Model file for the job. Use its own axes, mm. A direction names the side the tool comes from. Round coordinates to 2 decimals unless told otherwise and drop trailing zeros. Loops run counter-clockwise (first coordinate to the right, second up) from the corner with the lowest first, then second, coordinate; pieces in that order, holes last. Notation, with made-up numbers: M 32,47.5 L 43,47.5 A13 cw 43,58.5 Z; hole C 59,-34 d8. An arc over 180 degrees is marked long. Answer in a Markdown table with one row per item.
from build123d import *

# Parameters (mm, degrees)
ESQUISSE1_R             = 8.5
BOSS_EXTRU_1_DEPTH      = 7
ESQUISSE2_W             = 6
ESQUISSE2_H             = 2.6
ENL_V_MAT_EXTRU_1_DEPTH = 14.910427743
ESQUISSE7_R             = 2.95
ENL_V_MAT_EXTRU_8_DEPTH = 21.087060672
ESQUISSE9_R             = 4
BOSS_EXTRU_2_DEPTH      = 7
ENL_V_MAT_EXTRU_9_DEPTH = 19.45264218


with BuildPart() as part:
    # Esquisse1 → Boss.-Extru.1 (new body)
    with BuildSketch(Plane.XY):
        Circle(ESQUISSE1_R)
    extrude(amount=BOSS_EXTRU_1_DEPTH)

    # Esquisse2 → Enlèv. mat.-Extru.1 (cut, through all)
    with BuildSketch(Plane(origin=(0, 0, 0), x_dir=(-1, 0, 0), z_dir=(0, 0, -1))):
        with Locations((0, 4)):
            Rectangle(ESQUISSE2_W, ESQUISSE2_H)
    extrude(amount=-ENL_V_MAT_EXTRU_1_DEPTH, mode=Mode.SUBTRACT)

    # Enlèv. mat.-Extru.2: read off the stored shape, not the designer's step
    # Enlèv. mat.-Extru.2 outline → Enlèv. mat.-Extru.2 (revolve, cut)
    with BuildSketch(Plane.XY.offset(3.5)):
        Polygon((0, 5.3), (1.554616831, 5.3), (1.498760014, 8.500034923), (0, 8.500034923), align=None)
        Polygon((1.6, 2.7), (0, 2.7), (0, 0.7), (1.56508987, 0.7), align=None)
    revolve(axis=Axis((0, 0, 3.5), (0, 1, 0)), mode=Mode.SUBTRACT)

    # Esquisse7 → Enlèv. mat.-Extru.8 (cut, through all)
    with BuildSketch(Plane(origin=(0, 8.3, 0), x_dir=(1, 0, 0), z_dir=(0, 1, 0))):
        with Locations((0, -3.5)):
            Circle(ESQUISSE7_R)
    extrude(amount=ENL_V_MAT_EXTRU_8_DEPTH, mode=Mode.SUBTRACT)

    # Chanfrein1: read off the stored shape, not the designer's step
    # Chanfrein1 outline → Chanfrein1 (revolve, cut)
    with BuildSketch(Plane.XY.offset(3.5)):
        Polygon((2.95, 6.747748364), (2.95, 8.3), (1.502251636, 8.3), (1.553718474, 5.351466838), align=None)
    revolve(axis=Axis((0, 0, 3.5), (0, 1, 0)), mode=Mode.SUBTRACT)

    # Esquisse9 → Boss.-Extru.2 (add)
    with BuildSketch(Plane.XY.offset(7)):
        with Locations(Location((0, -1, 0), (0, 0, 112.331645009))):
            Circle(ESQUISSE9_R)
    extrude(amount=BOSS_EXTRU_2_DEPTH)

    # Esquisse10 → Enlèv. mat.-Extru.9 (cut, through all)
    with BuildSketch(Plane(origin=(0, 0, 0), x_dir=(-1, 0, 0), z_dir=(0, 0, -1))):
        with BuildLine():
            Line((-1.549193338, 2.15), (1.549193338, 2.15))
            ThreePointArc((1.549193338, 2.15), (0, -2.65), (-1.549193338, 2.15))
        make_face()
    extrude(amount=-ENL_V_MAT_EXTRU_9_DEPTH, mode=Mode.SUBTRACT)


solid = part.part
1. Wall check: probe 1 along Z at (x, y) = (0, 7.6); probe 2 along Y at (x, z) = (0, 11.25); probe 3 along Y at (x, z) = (-0.25, 1.5). Give the ranges that are in metal, low to high.
Verdict:
| item | result |
|---|---|
| probe 1 | z = 0 to 0.55, 6.45 to 7 |
| probe 2 | y = -5 to -2.65, 2.15 to 3 |
| probe 3 | y = -8.5 to -2.64, 2.15 to 2.7, 5.3 to 5.81 |
2. Tool access for faces 1 (the flat face through (0, 2.15, 1)), 2 (the cylindrical face through (3.94, -0.32, 10.45)), 3 (the conical face through (0.736, 2.414, 4.915)): list every direction of +Z, -Z, +X, -X, +Y, -Y with a clear straight run to the whole face (end or side of a thin tool).
Verdict:
| item | result |
|---|---|
| face 1 | +Z, -Z |
| face 2 | +Z |
| face 3 | none |
3. Pin check, flat tips, straight feed: pin 1 (2 mm diameter, centred on y = 4, z = 4.5, fed in from +X); pin 2 (4 mm diameter, centred on y = -2, z = 8, fed in from -X); pin 3 (0.8 mm diameter, centred on y = 4.5, z = 4.5, fed in from -X). Stop position of each tip, or through.
Verdict:
| item | result |
|---|---|
| pin 1 | stops at x = 7.95 |
| pin 2 | stops at x = -8.5 |
| pin 3 | stops at x = -7.45 |
4. Saw through at C-C (z = 13). Write the cut outline in (x, y), and give its area (3 significant figures).
Verdict:
| item | result |
|---|---|
| outline | C 0,-1 d8; hole M -1.55,2.15 A2.65 ccw long 1.55,2.15 Z |
| area | 29.3 mm² |
5. Saw through at B-B (x = 3.75). Write the cut outline in (y, z), and give its area (3 significant figures).
Verdict:
| item | result |
|---|---|
| outline | M -7.63,0 L 7.63,0 L 7.63,7 L 0.39,7 L 0.39,14 L -2.39,14 L -2.39,7 L -7.63,7 Z |
| area | 126 mm² |
6. Saw through at D-D (y = -4.25). Write the cut outline in (x, z), and give its area (3 significant figures).
Verdict:
| item | result |
|---|---|
| outline | M -7.36,0 L 7.36,0 L 7.36,7 L 2.33,7 L 2.33,14 L -2.33,14 L -2.33,7 L -7.36,7 Z |
| area | 136 mm² |
7. Mould opens along Z. For faces 4 (the flat face through (-2, -2, 0)), 5 (the flat face through (1, -3, 14)), 6 (the flat face through (1, 2.7, 2)), 7 (the cylindrical face through (1.36, 7.44, 6.12)) say: +Z half, -Z half, draft (parallel to the pull), parting line (faces both ways), or undercut.
Verdict:
| item | result |
|---|---|
| face 4 | -Z half |
| face 5 | +Z half |
| face 6 | draft |
| face 7 | undercut |
8. Saw through at A-A (y = -1). Write the cut outline in (x, z).
Verdict:
| item | result |
|---|---|
| outline | M -8.44,0 L -2.45,0 L -2.45,14 L -4,14 L -4,7 L -8.44,7 Z; M 2.45,0 L 8.44,0 L 8.44,7 L 4,7 L 4,14 L 2.45,14 Z |
